Geometry check sheet. Reference: the model listing, model coordinates, mm. A direction names the side the tool comes from. Round coordinates to 2 decimals unless told otherwise and drop trailing zeros. Write each loop counter-clockwise with the first axis right and the second up, starting at its lowest first coordinate (ties: lowest second). Pieces come first, ordered by that corner, then holes.
from build123d import *

# Parameters (mm, degrees)
SKETCH1_R           = 7.5
BOSS_EXTRUDE2_DEPTH = 14
CUT_EXTRUDE1_REACH  = 19.564
SKETCH2_R           = 4.25
BOSS_EXTRUDE3_START = -7.279118874
BOSS_EXTRUDE3_DEPTH = 1.03527618
FILLET1_R           = 10
CIRPATTERN1_COUNT   = 2
FILLET3_R           = 10


with BuildPart() as part:
    # Sketch1 → Boss-Extrude2 (new body)
    with BuildSketch(Plane(origin=(0, 0, 0), x_dir=(1, 0, 0), z_dir=(0, 1, 0))):
        with Locations(Location((0, 0, 0), (0, 0, 270))):
            Circle(SKETCH1_R)
    extrude(amount=BOSS_EXTRUDE2_DEPTH)

    # Sketch2 → Cut-Extrude1 (cut, up to next)
    with BuildSketch(Plane(origin=(0, 14, 0), x_dir=(1, 0, 0), z_dir=(0, 1, 0)), mode=Mode.PRIVATE) as cut_extrude1_sk1:
        with Locations(Location((0, 0, 0), (0, 0, 270))):
            Circle(SKETCH2_R)
    cut_extrude1_tool1 = extrude(cut_extrude1_sk1.sketch, amount=-CUT_EXTRUDE1_REACH, mode=Mode.PRIVATE) & part.part
    add(cut_extrude1_tool1.solids().sort_by_distance((0, 14, 0))[0], mode=Mode.SUBTRACT)

    # Boss-Extrude3: read off the stored shape, not the designer's step
    # Boss-Extrude3 outline → Boss-Extrude3 (add)
    with BuildSketch(Plane(origin=(0, 0, 0), x_dir=(0.9659258262890672, 0.2588190451025251, 0), z_dir=(0.25881904510252507, -0.9659258262890672, 0)).offset(BOSS_EXTRUDE3_START)):
        with BuildLine():
            add(Edge.make_bspline(
                [(-5.688266684, 1.344969698), (-4.547659305, 7.389056985), (1.811733316, 7.498803292)],
                knots=[0.18030465, 0.18030465, 0.18030465, 1.551469461, 1.551469461, 1.551469461], degree=2, weights=[1, 0.771122328, 0.993637519]))
            add(Edge.make_bspline(
                [(1.811733316, 7.498803292), (8.171125936, 7.389056985), (9.311733316, 1.344969698)],
                knots=[1.590123193, 1.590123193, 1.590123193, 2.961288004, 2.961288004, 2.961288004], degree=2, weights=[0.993637519, 0.771122328, 1]))
            Line((9.311733316, 1.344969698), (9.311733316, 94.5))
            Line((9.311733316, 94.5), (-5.688266684, 94.5))
            Line((-5.688266684, 94.5), (-5.688266684, 1.344969698))
        make_face()
    boss_extrude3 = extrude(amount=BOSS_EXTRUDE3_DEPTH)

    # Fillet1
    fillet1_edges = [part.edges().sort_by_distance(p)[0] for p in [
        (-7.244443697, 5.058857162, 94.5),
    ]]
    fillet(fillet1_edges, radius=FILLET1_R)

    # CirPattern1: Boss-Extrude3 ×2 about axis
    cirpattern1_axis = Axis((0, 0, 0), (0, 1, 0))
    for i in range(1, CIRPATTERN1_COUNT):
        add(boss_extrude3.rotate(cirpattern1_axis, i * 360 / CIRPATTERN1_COUNT))

    # Fillet3
    fillet3_edges = [part.edges().sort_by_distance(p)[0] for p in [
        (7.244443697, 5.058857162, -94.5),
    ]]
    fillet(fillet3_edges, radius=FILLET3_R)


solid = part.part
1. Depth check by flat-ended pin: pin 1 Ø8 at (x, z) = (3, 47.5) entering from -Y; pin 2 Ø5 at (y, z) = (8, 6) entering from -X; pin 3 Ø2 at (x, z) = (3, -14) entering from +Y. Enter the tip coordinate at first touch or a pass-through.
2. Access from +Z, -Z, +X, -X, +Y, -Y to the whole of each face (thin tool, end or side, straight path). Record for faces 1 (the face through (-3.2, 0, 3.2)), 2 (the face through (2.253, 6.902, 7.154)).
3. Release check for a two-part mould opening along X. For faces 3 (the face through (-4.49, 5.79, 91.49)), 4 (the face through (-3.2, 14, 3.2)), 5 (the face through (4.214, 7.098, -0.553)) record: +X half, -X half, draft (parallel to the pull), parting line (faces both ways), or undercut.
4. Scan lines: line 1 along X through (y, z) = (4.5, 0); line 2 along Z through (x, y) = (0.5, 4.5); line 3 along Y through (x, z) = (3.5, 43.5). Record each from-to range of solid material in increasing order.
5. Section check A-A (z = -19). Record the cut outline in (x, y).
Results below:
1. pin 1: stops at y = 6.2
1. pin 2: stops at x = -7.38
1. pin 3: stops at y = 7
2. face 1: +Z, -Z, +X, -X, -Y
2. face 2: none
3. face 3: -X half
3. face 4: draft
3. face 5: undercut
4. line 1: x = -7.5 to -4.25, 4.25 to 7.5
4. line 2: z = -7.48 to -4.22, 4.22 to 7.48
4. line 3: y = 7.4 to 8.47
5. outline: (-7.38, 8.44) - (7.11, 4.56) - (7.38, 5.56) - (-7.11, 9.44) - close
